Build history of the part. All positions in model axes, mm. Face numbers are marked on the shaded views. A direction names the side the tool comes from. Coordinates: 2 decimals unless noted, no trailing zeros. Loops run counter-clockwise (first coordinate to the right, second up) from the corner with the lowest first, then second, coordinate; pieces in that order, holes last. Notation, with made-up numbers: (54, 45.25) - (94, 45.25) arc R32 ccw to (94, 76.25) - close; hole circle Ø4 at (-15, -5.5). An arc over 180 degrees is marked (long way). One line per item, written item: value.
```python
from build123d import *

# Parameters (mm, degrees)
SKETCH2_R               = 63.5
BOSS_EXTRUDE1_DEPTH     = 9.525
SKETCH2_3_R             = 38.1
BOSS_EXTRUDE2_DEPTH     = 50.8
CUT_EXTRUDE1_DEPTH      = 50.8
CUT_EXTRUDE1_DEPTH_BACK = 50.8
SKETCH2_4_R             = 25.4
SKETCH3_R               = 3.175
CUT_EXTRUDE2_DEPTH      = 50.8


with BuildPart() as part:
    # Sketch2 → Boss-Extrude1 (new body)
    with BuildSketch(Plane(origin=(0, 0, 0), x_dir=(1, 0, 0), z_dir=(0, 1, 0))):
        with Locations(Location((0, 0, 0), (0, 0, 270))):
            Circle(SKETCH2_R)
    extrude(amount=-BOSS_EXTRUDE1_DEPTH)

    # Sketch2_3 → Boss-Extrude2 (add)
    with BuildSketch(Plane(origin=(0, 0, 0), x_dir=(1, 0, 0), z_dir=(0, 1, 0))):
        with Locations(Location((0, 0, 0), (0, 0, 270))):
            Circle(SKETCH2_3_R)
    extrude(amount=BOSS_EXTRUDE2_DEPTH)

    # Sketch2_4 → Cut-Extrude1 (cut, two sides: drawn at the far end of the back side and taken through both)
    with BuildSketch(Plane(origin=(0, 0, 0), x_dir=(1, 0, 0), z_dir=(0, 1, 0)).offset(-CUT_EXTRUDE1_DEPTH_BACK)):
        with Locations(Location((0, 0, 0), (0, 0, 270))):
            Circle(SKETCH2_4_R)
    extrude(amount=CUT_EXTRUDE1_DEPTH + CUT_EXTRUDE1_DEPTH_BACK, mode=Mode.SUBTRACT)

    # Sketch3 → Cut-Extrude2 (cut)
    with BuildSketch(Plane(origin=(0, -9.525, 0), x_dir=(-1, 0, 0), z_dir=(0, -1, 0))):
        with Locations(Location((0, -50.8, 0), (0, 0, 90))):
            Circle(SKETCH3_R)
        with Locations(Location((-50.8, 0, 0), (0, 0, 90))):
            Circle(SKETCH3_R)
        with Locations(Location((0, 50.8, 0), (0, 0, 90))):
            Circle(SKETCH3_R)
        with Locations(Location((50.8, 0, 0), (0, 0, 90))):
            Circle(SKETCH3_R)
    extrude(amount=-CUT_EXTRUDE2_DEPTH, mode=Mode.SUBTRACT)


solid = part.part
```
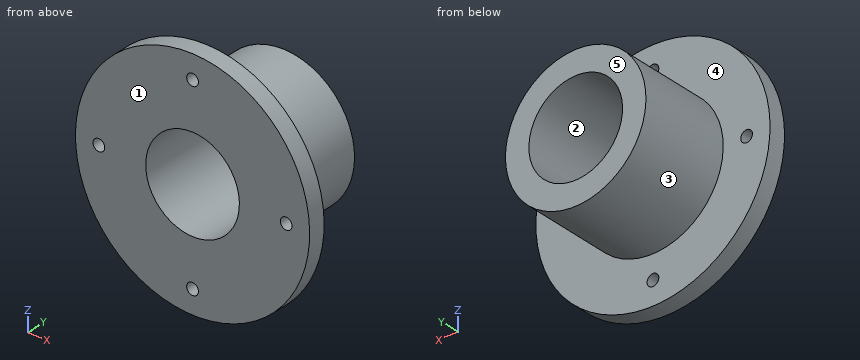
Item 1: Cut at A-A, the plane z = 50.8. Write the cut outline in (x, y) (3 decimals).
Check result:
outline: (-38.1, -9.525) - (-3.175, -9.525) - (-3.175, 0) - (-38.1, 0) - close; (3.175, -9.525) - (38.1, -9.525) - (38.1, 0) - (3.175, 0) - close
Item 2: Drop flat-ended pins along their axis: P1, Ø4, axis at x = 0, z = -50.8, coming from the -Y side; P2, Ø8.5, axis at x = -50.8, z = 0, coming from the +Y side; P3, Ø1.5, axis at y = 17, z = -24, coming from the +X side; P4, Ø3, axis at x = 11.5, y = 13, coming from the -Z side. Give the stop position or say it passes through.
Check result:
P1: passes through
P2: stops at y = 0
P3: stops at x = 30.18
P4: stops at z = -36.76
Item 3: Probe probe 1 along X at (y, z) = (-5, 0) (3 decimals); probe 2 along Y at (x, z) = (30, 47) (3 decimals); probe 3 along X at (y, z) = (5.5, 9). List the from-to ranges inside material, lowest first. Write a range as from..to.
Check result:
probe 1: x = -63.5..-53.975, -47.625..-25.4, 25.4..47.625, 53.975..63.5
probe 2: y = -9.525..0
probe 3: x = -37.02..-23.75, 23.75..37.02
Item 4: Cut at C-C, the plane z = 0. Write the cut outline in (x, y) (3 decimals), then the cut area to 3 significant figures.
Check result:
outline: (-63.5, -9.525) - (-53.975, -9.525) - (-53.975, 0) - (-63.5, 0) - close; (-47.625, -9.525) - (-25.4, -9.525) - (-25.4, 50.8) - (-38.1, 50.8) - (-38.1, 0) - (-47.625, 0) - close; (25.4, -9.525) - (47.625, -9.525) - (47.625, 0) - (38.1, 0) - (38.1, 50.8) - (25.4, 50.8) - close; (53.975, -9.525) - (63.5, -9.525) - (63.5, 0) - (53.975, 0) - close
area: 1,900 mm^2
Item 5: Cut at B-B, the plane x = 0. Write the cut outline in (y, z) (3 decimals), then the cut area to 3 significant figures.
Check result:
outline: (-9.525, -63.5) - (0, -63.5) - (0, -53.975) - (-9.525, -53.975) - close; (-9.525, -47.625) - (0, -47.625) - (0, -38.1) - (50.8, -38.1) - (50.8, -25.4) - (-9.525, -25.4) - close; (-9.525, 25.4) - (50.8, 25.4) - (50.8, 38.1) - (0, 38.1) - (0, 47.625) - (-9.525, 47.625) - close; (-9.525, 53.975) - (0, 53.975) - (0, 63.5) - (-9.525, 63.5) - close
area: 1,900 mm^2
Item 6: Pull direction X, two halves, no side cores. Call the marked faces 1, 2 and 3: released by +X, released by -X, zero draft, split by the parting line, or undercut.
Check result:
face 1: zero draft
face 2: undercut
face 3: split by the parting line
Item 7: Tool access for the marked faces 4 and 5: list every direction of +Z, -Z, +X, -X, +Y, -Y with a clear straight run to the whole face (end or side of a thin tool).
Check result:
face 4: +Y
face 5: +Z, -Z, +X, -X, +Y
Item 8: Cut at D-D, the plane x = 50.8. Write the cut outline in (y, z) (3 decimals).
Check result:
outline: (-9.525, -38.1) - (0, -38.1) - (0, -3.175) - (-9.525, -3.175) - close; (-9.525, 3.175) - (0, 3.175) - (0, 38.1) - (-9.525, 38.1) - close
